```python
from build123d import *

# Parameters (mm, degrees)
F1_DEPTH = 8.255
F2_R     = 2.0193
F3_DEPTH = 11.43


with BuildPart() as f1:
    # F0 (on Front) → F1 (new body, symmetric)
    with BuildSketch(Plane.XZ):
        Polygon((-12.7, 0), (0, 0), (0, 12.7), (-6.35, 12.7), (-12.7, 12.3672106016), align=None)
    extrude(amount=F1_DEPTH, both=True)

    # F2 (on face) → F3 (cut)
    with BuildSketch(Plane(origin=(0, 0, 0), x_dir=(1, 0, 0), z_dir=(0, 0, -1))):
        with Locations((-6.35, 0)):
            Circle(F2_R)
    extrude(amount=-F3_DEPTH, mode=Mode.SUBTRACT)


solid = f1.part
```
Input: part model. Units: mm. Frame: model coordinates. Coordinates: 2 decimals unless noted, no trailing zeros. Loops run counter-clockwise (first coordinate to the right, second up) from the corner with the lowest first, then second, coordinate; pieces in that order, holes last. Notation, with made-up numbers: M 65,-9.5 L 114,-9.5 A22 ccw 114,20.5 Z; hole C -4.5,-6.5 d6. An arc over 180 degrees is marked long. Use a Markdown table: item, result. Add a question column.
1) Section D-D, the plane x = -5. Return the cut outline in (y, z) (3 decimals), plus the area to 3 significant figures.
2) Section B-B, the plane y = 0. Return the cut outline in (x, z).
3) Draft query along X for faces 1 (the flat face through (-6, 8.255, 6)), 2 (the cylindrical face through (-4.424, -0.607, 5.635)), 3 (the flat face through (-6, 0, 11.43)), 4 (the flat face through (-9.481, -0.116, 12.536)). Return one class per face: +X half, -X half, draft (parallel to the pull), parting line (faces both ways), or undercut.
4) Pin query (flat end, axial travel): P1, Ø2.5, axis at x = -6.35, y = 0, coming from the -Z side. Return the tip coordinate at first contact, or that it passes through.
5) Section C-C, the plane x = -6.75. Return the cut outline in (y, z) (3 decimals), plus the area to 3 significant figures.
6) Section A-A, the plane z = 3.75. Return the cut outline in (x, y) (3 decimals), plus the area to 3 significant figures.
7) Line query: L1, parallel to X at y = 0, z = 5.25; L2, parallel to Y at x = -6.35, z = 4.5 (3 decimals); L3, parallel to Z at x = -6.5, y = -3. Output: solid intervals per line, ascending. Write a range as from..to.
Answer below:
| question | item | result |
|---|---|---|
| 1 | outline | M -8.255,0 L -1.502,0 L -1.502,11.43 L 1.502,11.43 L 1.502,0 L 8.255,0 L 8.255,12.7 L -8.255,12.7 Z |
| 1 | area | 175 mm2 |
| 2 | outline | M -12.7,0 L -8.37,0 L -8.37,11.43 L -4.33,11.43 L -4.33,0 L 0,0 L 0,12.7 L -6.35,12.7 L -12.7,12.37 Z |
| 3 | face 1 | draft |
| 3 | face 2 | undercut |
| 3 | face 3 | undercut |
| 3 | face 4 | -X half |
| 4 | P1 | z = 11.43 |
| 5 | outline | M -8.255,0 L -1.979,0 L -1.979,11.43 L 1.979,11.43 L 1.979,0 L 8.255,0 L 8.255,12.679 L -8.255,12.679 Z |
| 5 | area | 164 mm2 |
| 6 | outline | M -12.7,-8.255 L 0,-8.255 L 0,8.255 L -12.7,8.255 Z; hole C -6.35,0 d4.039 |
| 6 | area | 197 mm2 |
| 7 | L1 | -12.7..-8.37, -4.33..0 |
| 7 | L2 | -8.255..-2.019, 2.019..8.255 |
| 7 | L3 | 0..12.69 |
